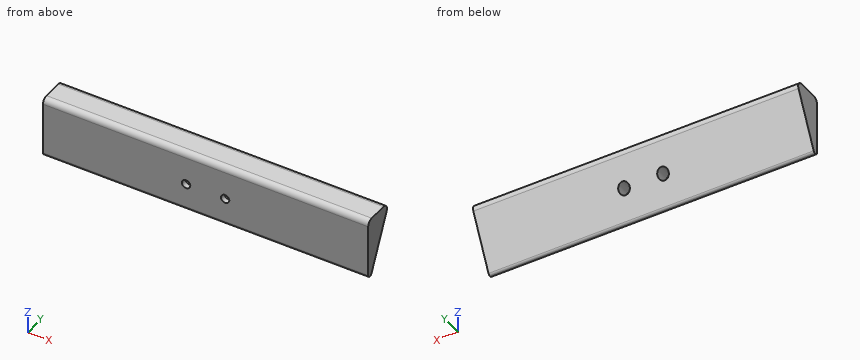
```python
from build123d import *

# Parameters (mm, degrees)
BOSS_EXTRUDE1_DEPTH = 116.65
SKETCH2_R           = 2
CUT_EXTRUDE1_DEPTH  = 8
SKETCH3_R           = 1.5
CUT_EXTRUDE2_DEPTH  = 119.961552208


with BuildPart() as part:
    # Sketch1 → Boss-Extrude1 (new body)
    with BuildSketch(Plane(origin=(0, 0, 0), x_dir=(0, 0, -1), z_dir=(1, 0, 0))):
        with BuildLine():
            Line((2, 0), (20.605762563, 0))
            ThreePointArc((20.605762563, 0), (21.580832575, 0.778102566), (21.03849363, 1.901523057))
            Line((21.03849363, 1.901523057), (2.865462135, 10.624578175))
            ThreePointArc((2.865462135, 10.624578175), (0.934853125, 10.514299657), (0, 8.82153206))
            Line((0, 8.82153206), (0, 2))
            ThreePointArc((0, 2), (0.585786438, 0.585786438), (2, 0))
        make_face()
    extrude(amount=BOSS_EXTRUDE1_DEPTH)

    # Sketch2 → Cut-Extrude1 (cut)
    with BuildSketch(Plane(origin=(0, 10, 0), x_dir=(1, 0, 0), z_dir=(0, 1, 0))):
        with Locations(Location((51.325, 11.951977883, 0), (0, 0, 270))):
            Circle(SKETCH2_R)
        with Locations(Location((65.325, 11.951977883, 0), (0, 0, 270))):
            Circle(SKETCH2_R)
    extrude(amount=-CUT_EXTRUDE1_DEPTH, mode=Mode.SUBTRACT)

    # Sketch3 → Cut-Extrude2 (cut, through all)
    with BuildSketch(Plane(origin=(0, 2, 0), x_dir=(1, 0, 0), z_dir=(0, 1, 0))):
        with Locations(Location((51.325, 11.951977883, 0), (0, 0, 270))):
            Circle(SKETCH3_R)
        with Locations(Location((65.325, 11.951977883, 0), (0, 0, 270))):
            Circle(SKETCH3_R)
    extrude(amount=-CUT_EXTRUDE2_DEPTH, mode=Mode.SUBTRACT)


solid = part.part
```
Geometry check sheet. Reference: the model listing, model coordinates, mm. Coordinates: 2 decimals unless noted, no trailing zeros. Loops run counter-clockwise (first coordinate to the right, second up) from the corner with the lowest first, then second, coordinate; pieces in that order, holes last.
Item 1: Sectioned sample at A-A, the plane x = 72. Record the boundary of the cut face in (y, z), then the cut area to 3 significant figures.
Item 2: Sectioned sample at B-B, the plane z = -17.5. Record the boundary of the cut face in (x, y), then the cut area to 3 significant figures.
Item 3: Sectioned sample at C-C, the plane y = 5.5. Record the boundary of the cut face in (x, z) (3 decimals).
Item 4: Thickness scan on line 1 (Z direction, x = 66, y = 3.5); line 2 (Z direction, x = 93, y = 9.25); line 3 (Y direction, x = 87.5, z = -19.25). Record the ranges inside material, lowest first.
Item 5: Go/stop test with flat-tipped pins: pin 1 Ø5 at (x, z) = (51, -17) entering from +Y; pin 2 Ø3.5 at (x, z) = (51.32, -11.95) entering from +Y; pin 3 Ø2 at (x, z) = (94, -18) entering from +Y. Record where each tip stops, or that it passes through.
Check result:
1. outline: (0, -20.61) arc R1 ccw to (1.9, -21.04) - (10.62, -2.87) arc R2 ccw to (8.82, 0) - (2, 0) arc R2 ccw to (0, -2) - close
1. area: 144 mm2
2. outline: (0, 0) - (116.65, 0) - (116.65, 3.6) - (0, 3.6) - close
2. area: 420 mm2
3. outline: (0, -13.542) - (50.111, -13.542) arc R2 cw (long way) to (52.539, -13.542) - (64.111, -13.542) arc R2 cw (long way) to (66.539, -13.542) - (116.65, -13.542) - (116.65, 0) - (0, 0) - close
4. line 1: z = -17.71 to -13.83, -10.07 to 0
4. line 2: z = -5.73 to -0.05
4. line 3: y = 0 to 2.76
5. pin 1: stops at y = 5.04
5. pin 2: stops at y = 2
5. pin 3: stops at y = 3.84
